For this review, take the finished solid that the model builds, in its own axes (mm). A direction names the side the tool comes from. Coordinates: 2 decimals unless noted, no trailing zeros. Order: outer loops, then holes, each group sorted by start corner. A loop starts at its lowest first (then second) coordinate and runs counter-clockwise, first axis right, second up. Notation, with made-up numbers: (15.5, 77.5) -> (34.5, 77.5) arc R18 cw to (34.5, 98.5) -> close; hole circle Ø11 at (61.25, -28). An arc over 180 degrees is marked (long way). Return JSON: item names as keys, results as strings. Group by question number.
Item 1: Take a section at D-D (z = 50). Write out the cut boundary in (x, y).
Item 2: Take a section at A-A (y = 15). Write out the cut boundary in (x, z).
Item 3: Machinability: for faces 1 (the flat face through (-131, 0, 84)), 2 (the flat face through (-131, 85, 185)), 3 (the cylindrical face through (-123.15, 116.99, 101.4)), which of the approach directions +Z, -Z, +X, -X, +Y, -Y give a long, thin tool a straight path to every point of the face, cutting with its end or side? Answer none if there is none.
Item 4: Take a section at C-C (y = 41). Write out the cut boundary in (x, z), then the cut area to 3 significant figures.
Item 5: Draft analysis for pull direction Z (two halves, no side actions). For faces 4 (the cylindrical face through (-132.99, 127.15, 101.4)), 5 (the cylindrical face through (-29.484, 125.07, 187.813)), 6 (the flat face through (-64, 123, 200)), state which applies: +Z half, -Z half, draft (parallel to the pull), parting line (faces both ways), or undercut.
Item 6: Take a section at B-B (z = 140). Write out the cut boundary in (x, y).
Item 7: Insertion check: pin 1 (3 mm diameter, centred on x = -130, z = 185.5, fed in from -Y); pin 2 (8 mm diameter, centred on x = -29.072, z = 190.953, fed in from -Y); pin 3 (5 mm diameter, centred on x = -132.5, y = 37, fed in from +Z). Each pin has a flat end and moves straight along its axis. Give the tip position at first contact, or say it passes through.
Item 8: For line 1 along X through (y, z) = (101.5, 109); line 2 along Y through (x, z) = (-127, 30); line 3 along Z through (x, y) = (0.5, 36.5), list the stretches that pass through material, from the lowest coordinate up.
```python
from build123d import *

# Parameters (mm, degrees)
SALIENTE_EXTRUIR1_DEPTH = 200
REDONDEO1_R             = 10
CROQUIS2_R              = 6
CORTAR_EXTRUIR1_DEPTH   = 147
CROQUIS3_W              = 30
CROQUIS3_H              = 85
CORTAR_EXTRUIR2_DEPTH   = 147
CORTAR_EXTRUIR3_REACH   = 132
CROQUIS4_R              = 3.1665


with BuildPart() as part:
    # Croquis1 → Saliente-Extruir1 (new body)
    with BuildSketch(Plane.XY):
        Polygon((-136, 0), (-126, 0), (-126, 120), (0, 120), (0, 0), (10, 0), (10, 130), (-136, 130), align=None)
    extrude(amount=SALIENTE_EXTRUIR1_DEPTH)

    # Redondeo1
    redondeo1_edges = [part.edges().sort_by_distance(p)[0] for p in [
        (-136, 130, 100),
        (10, 130, 100),
        (0, 120, 100),
        (-126, 120, 100),
    ]]
    fillet(redondeo1_edges, radius=REDONDEO1_R)

    # Croquis2 → Cortar-Extruir1 (cut, through all)
    with BuildSketch(Plane(origin=(10, 0, 0), x_dir=(0, 0, -1), z_dir=(1, 0, 0))):
        with Locations((-140, 15)):
            Circle(CROQUIS2_R)
        with Locations((-30, 15)):
            Circle(CROQUIS2_R)
    extrude(amount=-CORTAR_EXTRUIR1_DEPTH, mode=Mode.SUBTRACT)

    # Croquis3 → Cortar-Extruir2 (cut, through all)
    with BuildSketch(Plane(origin=(10, 0, 0), x_dir=(0, 0, -1), z_dir=(1, 0, 0))):
        with Locations((-185, 42.5)):
            Rectangle(CROQUIS3_W, CROQUIS3_H)
    extrude(amount=-CORTAR_EXTRUIR2_DEPTH, mode=Mode.SUBTRACT)

    # Croquis4 → Cortar-Extruir3 (cut, up to next)
    with BuildSketch(Plane(origin=(0, 130, 0), x_dir=(1, 0, 0), z_dir=(0, 1, 0)), mode=Mode.PRIVATE) as cortar_extruir3_sk1:
        with Locations((-96.928, -190.953)):
            Circle(CROQUIS4_R)
    cortar_extruir3_tool1 = extrude(cortar_extruir3_sk1.sketch, amount=-CORTAR_EXTRUIR3_REACH, mode=Mode.PRIVATE) & part.part
    add(cortar_extruir3_tool1.solids().sort_by_distance((-96.928, 130, 190.953))[0], mode=Mode.SUBTRACT)
    # Croquis4 → Cortar-Extruir3 (cut, up to next)
    with BuildSketch(Plane(origin=(0, 130, 0), x_dir=(1, 0, 0), z_dir=(0, 1, 0)), mode=Mode.PRIVATE) as cortar_extruir3_sk2:
        with Locations((-29.072, -190.953)):
            Circle(CROQUIS4_R)
    cortar_extruir3_tool2 = extrude(cortar_extruir3_sk2.sketch, amount=-CORTAR_EXTRUIR3_REACH, mode=Mode.PRIVATE) & part.part
    add(cortar_extruir3_tool2.solids().sort_by_distance((-29.072, 130, 190.953))[0], mode=Mode.SUBTRACT)
    # Croquis4 → Cortar-Extruir3 (cut, up to next)
    with BuildSketch(Plane(origin=(0, 130, 0), x_dir=(1, 0, 0), z_dir=(0, 1, 0)), mode=Mode.PRIVATE) as cortar_extruir3_sk3:
        with Locations((-96.928, -102.741)):
            Circle(CROQUIS4_R)
    cortar_extruir3_tool3 = extrude(cortar_extruir3_sk3.sketch, amount=-CORTAR_EXTRUIR3_REACH, mode=Mode.PRIVATE) & part.part
    add(cortar_extruir3_tool3.solids().sort_by_distance((-96.928, 130, 102.741))[0], mode=Mode.SUBTRACT)
    # Croquis4 → Cortar-Extruir3 (cut, up to next)
    with BuildSketch(Plane(origin=(0, 130, 0), x_dir=(1, 0, 0), z_dir=(0, 1, 0)), mode=Mode.PRIVATE) as cortar_extruir3_sk4:
        with Locations((-29.072, -102.741)):
            Circle(CROQUIS4_R)
    cortar_extruir3_tool4 = extrude(cortar_extruir3_sk4.sketch, amount=-CORTAR_EXTRUIR3_REACH, mode=Mode.PRIVATE) & part.part
    add(cortar_extruir3_tool4.solids().sort_by_distance((-29.072, 130, 102.741))[0], mode=Mode.SUBTRACT)


solid = part.part
```
Findings below:
{
 "1": {"outline": "(-136, 0) -> (-126, 0) -> (-126, 110) arc R10 cw to (-116, 120) -> (-10, 120) arc R10 cw to (0, 110) -> (0, 0) -> (10, 0) -> (10, 120) arc R10 ccw to (0, 130) -> (-126, 130) arc R10 ccw to (-136, 120) -> close"},
 "2": {"outline": "(-136, 0) -> (-126, 0) -> (-126, 24) -> (-136, 24) -> close; (-136, 36) -> (-126, 36) -> (-126, 134) -> (-136, 134) -> close; (-136, 146) -> (-126, 146) -> (-126, 170) -> (-136, 170) -> close; (0, 0) -> (10, 0) -> (10, 24) -> (0, 24) -> close; (0, 36) -> (10, 36) -> (10, 134) -> (0, 134) -> close; (0, 146) -> (10, 146) -> (10, 170) -> (0, 170) -> close"},
 "3": {"face 1": "+Z, -Z, +X, -X, -Y", "face 2": "+Z, +X, -X, -Y", "face 3": "+Z, -Z, -Y"},
 "4": {"outline": "(-136, 0) -> (-126, 0) -> (-126, 170) -> (-136, 170) -> close; (0, 0) -> (10, 0) -> (10, 170) -> (0, 170) -> close", "area": "3,400 mm2"},
 "5": {"face 4": "draft", "face 5": "undercut", "face 6": "+Z half"},
 "6": {"outline": "(-136, 0) -> (-126, 0) -> (-126, 9) -> (-136, 9) -> close; (-136, 21) -> (-126, 21) -> (-126, 110) arc R10 cw to (-116, 120) -> (-10, 120) arc R10 cw to (0, 110) -> (0, 21) -> (10, 21) -> (10, 120) arc R10 ccw to (0, 130) -> (-126, 130) arc R10 ccw to (-136, 120) -> close; (0, 0) -> (10, 0) -> (10, 9) -> (0, 9) -> close"},
 "7": {"pin 1": "stops at y = 85", "pin 2": "stops at y = 120", "pin 3": "stops at z = 170"},
 "8": {"line 1": "x = -136 to -126, 0 to 10", "line 2": "y = 0 to 9, 21 to 129.95", "line 3": "z = 0 to 170"}
}
